Geometry check sheet. Reference: the model listing, model coordinates, mm. Give positions to 0.01 mm unless a question says otherwise; leave off trailing zeros. Loops run counter-clockwise (first coordinate to the right, second up) from the corner with the lowest first, then second, coordinate; pieces in that order, holes last. Notation, with made-up numbers: (57.5, 23) -> (94.5, 23) arc R20 ccw to (94.5, 47) -> close; hole circle Ø6 at (-21, 8.5). An arc over 180 degrees is marked (long way). Write each question's results on one line, items separated by ' | '. Start each with the question number.
1) Sectioned sample at A-A on x = 87. Record the cut outline in (y, z), then the cut area to 3 significant figures.
2) Sectioned sample at C-C on z = -129.5. Record the cut outline in (x, y).
3) Scan lines: line 1 (Z direction, x = 78, y = -5); line 2 (X direction, y = -2.5, z = 60); line 3 (X direction, y = -33.5, z = 85). Record each from-to range of solid material in increasing order. Write a range as from..to.
4) Sectioned sample at B-B on z = -14. Record the cut outline in (x, y), then the cut area to 3 significant figures.
5) Depth check by flat-ended pin: pin 1 (5 mm diameter, centred on x = -38, y = -13, fed in from -Z); pin 2 (4 mm diameter, centred on x = -66.5, y = -27, fed in from +Z); pin 3 (5 mm diameter, centred on x = -30.5, y = -26, fed in from -Z); pin 4 (2 mm diameter, centred on x = -10.5, z = 11, fed in from +Y). Enter the tip coordinate at first touch or a pass-through.
```python
from build123d import *

# Parameters (mm, degrees)
F1_DEPTH = 100
F2_SCALE = 0.3937


with BuildPart() as f1:
    # F0 (on Front) → F1 (new body)
    with BuildSketch(Plane.XZ):
        Polygon((-253.359285, -293.078281), (-254.4597146, -389.5920072), (182.3918882, -394.5729472), (183.49976, -394.5855964), (184.6076064, -394.5982202), (185.7154782, -394.610844), (186.8233246, -394.6234932), (187.9311964, -394.636117), (189.0390428, -394.6487408), (190.1469146, -394.66139), (191.254761, -394.6740138), (192.3626328, -394.6866376), (193.4705046, -394.6992868), (194.578351, -394.7119106), (195.6862228, -394.7245344), (196.7940692, -394.7371582), (197.901941, -394.7498074), (199.0098128, -394.7624312), (200.1176592, -394.775055), (201.2255056, -394.7877042), (202.3333774, -394.800328), (245.5105834, -395.2926308), (246.524145, -306.3983966), (203.346939, -305.9061192), (202.2390672, -305.89347), (201.1312208, -305.8808462), (200.0233744, -305.8682224), (198.9155026, -305.8555732), (197.8076308, -305.8429494), (196.6997844, -305.8303256), (195.5919126, -305.8176764), (194.4840662, -305.8050526), (193.3761944, -305.7924288), (192.2683226, -305.7797796), (191.1604762, -305.7671558), (190.0526044, -305.754532), (188.944758, -305.7418828), (187.8368862, -305.729259), (186.7290398, -305.7166352), (185.621168, -305.7040114), (184.5133216, -305.6913622), (183.4054498, -305.6787384), (183.4923178, -298.059221), (203.810997, -298.2908944), (203.9373366, -287.2123034), (204.0636508, -276.133687), (204.189965, -265.055096), (204.3162792, -253.9764796), (204.4425934, -242.8978886), (204.5689076, -231.8192722), (204.6952218, -220.7406812), (204.821536, -209.6620648), (204.9478756, -198.5834738), (205.0741898, -187.5048574), (205.200504, -176.4262664), (205.3268182, -165.34765), (205.4531324, -154.2690336), (205.5794466, -143.1904426), (205.7057608, -132.1118262), (205.832075, -121.0332352), (205.9583892, -109.9546442), (206.0847288, -98.8760278), (185.7660496, -98.6443544), (185.8529176, -91.0248624), (186.960764, -91.0374862), (188.0686358, -91.05011), (189.1765076, -91.0627338), (190.284354, -91.075383), (191.3922258, -91.0880068), (192.5000722, -91.1006306), (193.607944, -91.1132798), (194.7157904, -91.1259036), (195.8236368, -91.1385274), (196.9315086, -91.1511766), (198.0393804, -91.1638004), (199.1472522, -91.1764242), (200.2550986, -91.1890734), (201.3629704, -91.2016972), (202.4708168, -91.214321), (203.5786632, -91.2269702), (204.686535, -91.239594), (205.7944068, -91.2522178), (248.9715874, -91.7445206), (250.998736, 86.0439224), (207.82153, 86.5362252), (206.7136582, 86.548849), (205.6058118, 86.5614982), (204.49794, 86.574122), (203.3900936, 86.5867458), (202.2822218, 86.5993696), (201.1743754, 86.6120188), (200.0665036, 86.6246426), (198.9586318, 86.6372664), (197.8507854, 86.6499156), (196.742939, 86.6625394), (195.6350672, 86.6751632), (194.5271954, 86.6878124), (193.419349, 86.7004362), (192.3114772, 86.71306), (191.2036308, 86.7257092), (190.095759, 86.738333), (188.9879126, 86.7509568), (187.8800408, 86.7635806), (187.9669088, 94.383098), (208.285588, 94.1514246), (208.4119276, 105.2300156), (208.5382418, 116.308632), (208.664556, 127.3872484), (208.7908702, 138.4658394), (208.9171844, 149.5444304), (209.0434986, 160.6230468), (209.1698128, 171.7016632), (209.296127, 182.7802542), (209.4224412, 193.8588706), (209.5487808, 204.937487), (209.675095, 216.016078), (209.8014092, 227.094669), (209.9277234, 238.1732854), (210.0540376, 249.2518764), (210.1803518, 260.3304928), (210.306666, 271.4090838), (210.4329802, 282.4877002), (210.5593198, 293.5663166), (190.2406406, 293.7979646), (190.3275086, 301.417482), (191.435355, 301.4048582), (192.5432268, 301.392209), (193.6510986, 301.3795852), (194.758945, 301.3669614), (195.8668168, 301.3543122), (196.9746886, 301.3416884), (198.082535, 301.3290646), (199.1903814, 301.3164154), (200.2982532, 301.3037916), (201.4060996, 301.2911678), (202.5139714, 301.278544), (203.6218432, 301.2658948), (204.7296896, 301.253271), (205.8375614, 301.2406472), (206.9454078, 301.227998), (208.0532796, 301.2153742), (209.161126, 301.2027504), (210.2689978, 301.1901012), (253.4461784, 300.6977984), (254.45974, 389.5920326), (211.2825594, 390.0843354), (210.1746876, 390.0969592), (209.0668412, 390.109583), (207.9589694, 390.1222322), (206.851123, 390.134856), (205.7432512, 390.1474798), (204.6354048, 390.160129), (203.527533, 390.1727528), (202.4196612, 390.1853766), (201.3118148, 390.1980258), (200.2039684, 390.2106496), (199.0960966, 390.2232734), (197.9882502, 390.2359226), (196.8803784, 390.2485464), (195.7725066, 390.2611702), (194.6646602, 390.2738194), (193.5567884, 390.2864432), (192.4489166, 390.299067), (191.3410702, 390.3116908), (-245.5105326, 395.2926308), (-246.6109876, 298.7789046), (-246.7373018, 287.7003136), (-246.863616, 276.6216972), (-246.9899302, 265.5431062), (-247.1162444, 254.4644898), (-247.2425586, 243.3858988), (-247.3688728, 232.3072824), (-247.495187, 221.2286914), (-247.6215266, 210.150075), (-247.7478408, 199.071484), (-247.874155, 187.9928676), (-248.0004692, 176.9142766), (-248.1267834, 165.8356602), (-248.2530976, 154.7570438), (-248.3794118, 143.6784528), (-248.505726, 132.5998618), (-248.6320402, 121.5212454), (-248.7583798, 110.442629), (-248.884694, 99.364038), (-251.0855532, -93.6634144), (-251.2118928, -104.7420308), (-251.338207, -115.8206218), (-251.4645212, -126.8992128), (-251.5908354, -137.9778292), (-251.7171496, -149.0564202), (-251.8434638, -160.1350366), (-251.969778, -171.213653), (-252.0960922, -182.292244), (-252.2224318, -193.3708604), (-252.348746, -204.4494514), (-252.4750602, -215.5280678), (-252.6013744, -226.6066588), (-252.7276886, -237.6852752), (-252.8540028, -248.7638662), (-252.980317, -259.8424826), (-253.1066312, -270.9210736), (-253.2329454, -281.99969), align=None)
    extrude(amount=F1_DEPTH)


with BuildPart() as f1_1:
    # F2: moved
    add(f1.part.scale(F2_SCALE))


solid = f1_1.part
```
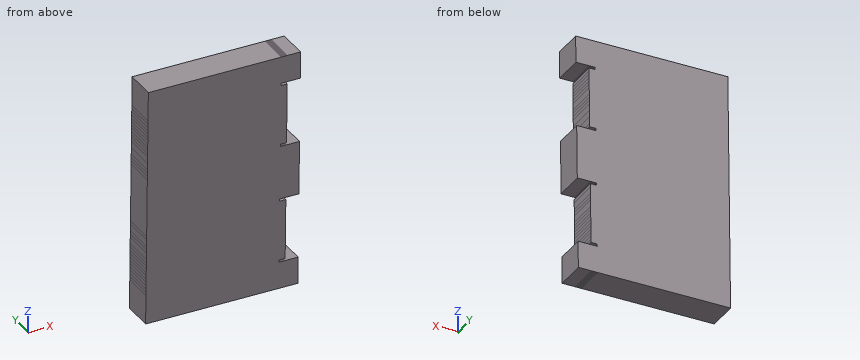
Result:
1) outline: (-39.37, -155.52) -> (0, -155.52) -> (0, -120.51) -> (-39.37, -120.51) -> close; (-39.37, -35.99) -> (0, -35.99) -> (0, 34.01) -> (-39.37, 34.01) -> close; (-39.37, 118.53) -> (0, 118.53) -> (0, 153.53) -> (-39.37, 153.53) -> close | area: 5,510 mm^2
2) outline: (-99.91, -39.37) -> (96.96, -39.37) -> (96.96, 0) -> (-99.91, 0) -> close
3) line 1: -155.41..-120.41, -117.41..-38.89, -35.89..34.11, 37.11..115.63, 118.63..153.64 | line 2: -97.75..82.26 | line 3: -97.46..82.55
4) outline: (-98.59, -39.37) -> (98.27, -39.37) -> (98.27, 0) -> (-98.59, 0) -> close | area: 7,750 mm^2
5) pin 1: z = -154.12 | pin 2: z = 155.31 | pin 3: z = -154.21 | pin 4: y = 0
